```python
from build123d import *

# Parameters (mm, degrees)
ESQUISSE1_W                  = 55
ESQUISSE1_H                  = 45
BOSS_EXTRU_1_DEPTH           = 12
ESQUISSE2_R                  = 4.25
ENL_V_MAT_EXTRU_1_DEPTH      = 55.085580333
ENL_V_MAT_EXTRU_2_DEPTH      = 12.25
ENL_V_MAT_EXTRU_2_DEPTH_BACK = 12.25
ESQUISSE3_R                  = 7.75
ESQUISSE4_R                  = 11
ENL_V_MAT_EXTRU_3_DEPTH      = 3
ESQUISSE5_R                  = 5
ENL_V_MAT_EXTRU_4_DEPTH      = 15
ENL_V_MAT_EXTRU_5_DEPTH      = 38.503333185
ENL_V_MAT_EXTRU_5_DEPTH_BACK = 38.503333185
ESQUISSE6_R                  = 1.5
ESQUISSE7_R                  = 2.5
ENL_V_MAT_EXTRU_6_DEPTH      = 4
CHANFREIN3_SIZE              = 5
ESQUISSE9_W                  = 60
ESQUISSE9_H                  = 18
BOSS_EXTRU_2_DEPTH           = 25
ESQUISSE10_W                 = 40.5
ESQUISSE10_H                 = 20
ENL_V_MAT_EXTRU_7_DEPTH      = 30
ESQUISSE11_R                 = 2.15
ENL_V_MAT_EXTRU_8_DEPTH      = 51.17220346
CONG_2_R                     = 5
CONG_3_R                     = 5
ESQUISSE12_W                 = 5
ESQUISSE12_H                 = 2
ENL_V_MAT_EXTRU_9_DEPTH      = 9
SYM_TRIE4_COPY_1_SKETCH_W    = 5
SYM_TRIE4_COPY_1_SKETCH_H    = 2
SYM_TRIE4_COPY_1_DEPTH       = 9
ESQUISSE13_W                 = 29
ESQUISSE13_H                 = 3
BOSS_EXTRU_3_DEPTH           = 25
BOSS_EXTRU_4_REACH           = 52.172
ESQUISSE14_W                 = 29
ESQUISSE14_H                 = 2.5
ESQUISSE15_R                 = 1.5
ENL_V_MAT_EXTRU_10_DEPTH     = 9
ENL_V_MAT_EXTRU_11_DEPTH     = 2


with BuildPart() as part:
    # Esquisse1 → Boss.-Extru.1 (new body)
    with BuildSketch(Plane.XY):
        Rectangle(ESQUISSE1_W, ESQUISSE1_H)
    extrude(amount=BOSS_EXTRU_1_DEPTH)

    # Esquisse2 → Enlèv. mat.-Extru.1 (cut, through all)
    with BuildSketch(Plane(origin=(0, 22.5, 0), x_dir=(1, 0, 0), z_dir=(0, 1, 0))):
        with Locations((-12.5, -12)):
            Circle(ESQUISSE2_R)
        with Locations((12.5, -12)):
            Circle(ESQUISSE2_R)
    extrude(amount=-ENL_V_MAT_EXTRU_1_DEPTH, mode=Mode.SUBTRACT)

    # Esquisse3 → Enlèv. mat.-Extru.2 (cut, two sides: drawn at the far end of the back side and taken through both)
    with BuildSketch(Plane(origin=(0, 0, 0), x_dir=(1, 0, 0), z_dir=(0, 1, 0)).offset(-ENL_V_MAT_EXTRU_2_DEPTH_BACK)):
        with Locations((-12.5, -12)):
            Circle(ESQUISSE3_R)
    extrude(amount=ENL_V_MAT_EXTRU_2_DEPTH + ENL_V_MAT_EXTRU_2_DEPTH_BACK, mode=Mode.SUBTRACT)

    # Esquisse4 → Enlèv. mat.-Extru.3 (cut)
    with BuildSketch(Plane(origin=(0, 7.5, 0), x_dir=(1, 0, 0), z_dir=(0, 1, 0))):
        with Locations((12.5, -12)):
            Circle(ESQUISSE4_R)
    enl_v_mat_extru_3 = extrude(amount=-ENL_V_MAT_EXTRU_3_DEPTH, mode=Mode.SUBTRACT)

    # Esquisse5 → Enlèv. mat.-Extru.4 (cut)
    with BuildSketch(Plane(origin=(0, 7.5, 0), x_dir=(1, 0, 0), z_dir=(0, 1, 0))):
        with Locations((12.5, -12)):
            Circle(ESQUISSE5_R)
    extrude(amount=-ENL_V_MAT_EXTRU_4_DEPTH, mode=Mode.SUBTRACT)

    # Esquisse6 → Enlèv. mat.-Extru.5 (cut, two sides: drawn at the far end of the back side and taken through both)
    with BuildSketch(Plane(origin=(0, 0, 0), x_dir=(-1, 0, 0), z_dir=(0, 0, -1)).offset(-ENL_V_MAT_EXTRU_5_DEPTH_BACK)):
        with Locations((23.5, -18.5)):
            Circle(ESQUISSE6_R)
        with Locations((-23.5, -18.5)):
            Circle(ESQUISSE6_R)
        with Locations((-23.5, 18.5)):
            Circle(ESQUISSE6_R)
        with Locations((23.5, 18.5)):
            Circle(ESQUISSE6_R)
    extrude(amount=ENL_V_MAT_EXTRU_5_DEPTH + ENL_V_MAT_EXTRU_5_DEPTH_BACK, mode=Mode.SUBTRACT)

    # Esquisse7 → Enlèv. mat.-Extru.6 (cut)
    with BuildSketch(Plane(origin=(0, 0, 0), x_dir=(-1, 0, 0), z_dir=(0, 0, -1))):
        with Locations((23.5, -18.5)):
            Circle(ESQUISSE7_R)
        with Locations(Location((23.5, 18.5, 0), (0, 0, 180))):
            Circle(ESQUISSE7_R)
        with Locations((-23.5, 18.5)):
            Circle(ESQUISSE7_R)
        with Locations(Location((-23.5, -18.5, 0), (0, 0, 180))):
            Circle(ESQUISSE7_R)
    extrude(amount=-ENL_V_MAT_EXTRU_6_DEPTH, mode=Mode.SUBTRACT)

    # Chanfrein3
    # the kernel refuses this chamfer: 5 mm, written as the material it takes off along each edge
    with BuildSketch(Plane(origin=(-27.5, 35.35841494, 0), x_dir=(0.9996219169112968, 0, -0.027495876610586372), z_dir=(0, -1, 0)), Plane(origin=(27.5, -35.35841494, 0), x_dir=(-0.9996219169112968, 0, -0.027495876610586372), z_dir=(0, 1, 0))) as chanfrein3_piece_1:
        Polygon((CHANFREIN3_SIZE * 0.999621916911, CHANFREIN3_SIZE * 0.0274958766106), (-CHANFREIN3_SIZE * 0.0274958766106, CHANFREIN3_SIZE * 0.999621916911), (0, 0), align=None)
    extrude(amount=70.71682988, mode=Mode.SUBTRACT)

    # Symétrie2: Enlèv. mat.-Extru.3 across plane
    add(enl_v_mat_extru_3.mirror(Plane.ZX), mode=Mode.SUBTRACT)

    # Esquisse9 → Boss.-Extru.2 (add)
    with BuildSketch(Plane(origin=(0, 0, 0), x_dir=(-1, 0, 0), z_dir=(0, 0, -1))):
        Rectangle(ESQUISSE9_W, ESQUISSE9_H)
    extrude(amount=BOSS_EXTRU_2_DEPTH)

    # Esquisse10 → Enlèv. mat.-Extru.7 (cut)
    with BuildSketch(Plane(origin=(0, 9, 0), x_dir=(1, 0, 0), z_dir=(0, 1, 0))):
        with Locations((0, 12.5)):
            Rectangle(ESQUISSE10_W, ESQUISSE10_H)
    extrude(amount=-ENL_V_MAT_EXTRU_7_DEPTH, mode=Mode.SUBTRACT)

    # Esquisse11 → Enlèv. mat.-Extru.8 (cut, through all)
    with BuildSketch(Plane(origin=(0, -9, 0), x_dir=(-1, 0, 0), z_dir=(0, -1, 0))):
        with Locations(Location((-23.65, 7.4, 0), (0, 0, 90))):
            Circle(ESQUISSE11_R)
        with Locations(Location((-23.65, 17.6, 0), (0, 0, 90))):
            Circle(ESQUISSE11_R)
        with Locations(Location((24.15, 7.4, 0), (0, 0, 90))):
            Circle(ESQUISSE11_R)
        with Locations(Location((24.15, 17.6, 0), (0, 0, 90))):
            Circle(ESQUISSE11_R)
    extrude(amount=-ENL_V_MAT_EXTRU_8_DEPTH, mode=Mode.SUBTRACT)

    # Congé2
    cong_2_edges = [part.edges().sort_by_distance(p)[0] for p in [
        (-30, 0, 0),
        (30, 0, 0),
    ]]
    fillet(cong_2_edges, radius=CONG_2_R)

    # Congé3
    cong_3_edges = [part.edges().sort_by_distance(p)[0] for p in [
        (-30, 0, -25),
        (30, 0, -25),
    ]]
    fillet(cong_3_edges, radius=CONG_3_R)

    # Esquisse12 → Enlèv. mat.-Extru.9 (cut)
    with BuildSketch(Plane(origin=(30, 0, 0), x_dir=(0, 0, -1), z_dir=(1, 0, 0))):
        with Locations((7.4, 4.5)):
            Rectangle(ESQUISSE12_W, ESQUISSE12_H)
        with Locations((17.6, 4.5)):
            Rectangle(ESQUISSE12_W, ESQUISSE12_H)
    enl_v_mat_extru_9 = extrude(amount=-ENL_V_MAT_EXTRU_9_DEPTH, mode=Mode.SUBTRACT)

    # Symétrie3: Enlèv. mat.-Extru.9 across plane
    add(enl_v_mat_extru_9.mirror(Plane(origin=(0, 0, 0), x_dir=(0, 0, 1), z_dir=(1, 0, 0))), mode=Mode.SUBTRACT)

    # Symétrie4: Enlèv. mat.-Extru.9 across plane
    add(enl_v_mat_extru_9.mirror(Plane.ZX), mode=Mode.SUBTRACT)

    # Symétrie4 copy 1 sketch → Symétrie4 copy 1 (cut)
    with BuildSketch(Plane(origin=(-30, 0, 0), x_dir=(0, 0, -1), z_dir=(-1, 0, 0))):
        with Locations((7.4, 4.5)):
            Rectangle(SYM_TRIE4_COPY_1_SKETCH_W, SYM_TRIE4_COPY_1_SKETCH_H)
        with Locations((17.6, 4.5)):
            Rectangle(SYM_TRIE4_COPY_1_SKETCH_W, SYM_TRIE4_COPY_1_SKETCH_H)
    extrude(amount=-SYM_TRIE4_COPY_1_DEPTH, mode=Mode.SUBTRACT)

    # Esquisse13 → Boss.-Extru.3 (add)
    with BuildSketch(Plane(origin=(0, 0, 0), x_dir=(-1, 0, 0), z_dir=(0, 0, -1))):
        with Locations((0, 21)):
            Rectangle(ESQUISSE13_W, ESQUISSE13_H)
    extrude(amount=BOSS_EXTRU_3_DEPTH)

    # Esquisse14 → Boss.-Extru.4 (add, up to next)
    with BuildSketch(Plane(origin=(0, 9, 0), x_dir=(1, 0, 0), z_dir=(0, 1, 0)), mode=Mode.PRIVATE) as boss_extru_4_sk1:
        with Locations((0, 23.75)):
            Rectangle(ESQUISSE14_W, ESQUISSE14_H)
    boss_extru_4_tool1 = extrude(boss_extru_4_sk1.sketch, amount=BOSS_EXTRU_4_REACH, mode=Mode.PRIVATE) - part.part
    add(boss_extru_4_tool1.solids().sort_by_distance((0, 9, -23.75))[0])

    # Esquisse15 → Enlèv. mat.-Extru.10 (cut)
    with BuildSketch(Plane(origin=(0, 22.5, 0), x_dir=(1, 0, 0), z_dir=(0, 1, 0))):
        with Locations(Location((-10.25, 12.5, 0), (0, 0, 270))):
            Circle(ESQUISSE15_R)
    extrude(amount=-ENL_V_MAT_EXTRU_10_DEPTH, mode=Mode.SUBTRACT)

    # Esquisse16 → Enlèv. mat.-Extru.11 (cut)
    with BuildSketch(Plane(origin=(0, 22.5, 0), x_dir=(1, 0, 0), z_dir=(0, 1, 0))):
        Polygon((-8.806624327, 15), (-11.693375673, 15), (-13.136751346, 12.5), (-11.693375673, 10), (-8.806624327, 10), (-7.363248654, 12.5), align=None)
    extrude(amount=-ENL_V_MAT_EXTRU_11_DEPTH, mode=Mode.SUBTRACT)


solid = part.part
```
Part model, mm, in its own coordinate system. A direction names the side the tool comes from. Round coordinates to 2 decimals unless told otherwise and drop trailing zeros. Write each loop counter-clockwise with the first axis right and the second up, starting at its lowest first coordinate (ties: lowest second). Pieces come first, ordered by that corner, then holes. Notation, with made-up numbers: M -19.75,73.25 L -6.75,73.25 A23 cw -6.75,90.25 Z; hole C -13,83.25 d5. An arc over 180 degrees is marked long. Answer as CSV lines item,"result". Start each with the question number.
1) Band-saw the part on C-C (x = -4). List the corners of the cut face in (y, z), then the cut area to 3 significant figures.
2) Drill centre lines: L1, parallel to Y at x = 23.5, z = 10.5; L2, parallel to X at y = 0.5, z = -7.4; L3, parallel to Y at x = -27, z = -19.5. Where is each one in solid material? Low to high.
3) Drop flat-ended pins along their axis: pin 1 (5.5 mm diameter, centred on x = 24, y = -17.5, fed in from -Z); pin 2 (5 mm diameter, centred on x = 12.5, y = -6, fed in from +Z); pin 3 (5.5 mm diameter, centred on x = 23.65, z = -7.4, fed in from +Y); pin 4 (2.5 mm diameter, centred on x = 24.5, z = -7.5, fed in from +Y). Give the stop position or say it passes through.
4) Band-saw the part on A-A (y = 14). List the corners of the cut face in (x, z), then the cut area to 3 significant figures.
5) Band-saw the part on B-B (y = 6.5). List the corners of the cut face in (x, z).
6) Which spindle directions (+Z, -Z, +X, -X, +Y, -Y) get a long thin tool onto all of the face, cutting with end or side? Do faces 1 (the face through (-22, 20, 4)), 2 (the face through (-27, 5.5, -18)), 3 (the face through (14.5, 20, -15)). Say none if no direction does.
7) Band-saw the part on D-D (y = 18.5). List the corners of the cut face in (x, z), then the cut area to 3 significant figures.
8) Mould opens along X. For faces 4 (the face through (-22.39, -17.49, 8.06)), 5 (the face through (-26, -4, -15.1)), 6 (the face through (-22.34, -0.05, -18.76)), 7 (the face through (27.5, 0, 8)) say: +X half, -X half, draft (parallel to the pull), parting line (faces both ways), or undercut.
Worked out:
1,outline,"M -22.5,0 L -9,0 L -9,-2.5 L 9,-2.5 L 9,0 L 19.5,0 L 19.5,-22.5 L -9,-22.5 L -9,-25 L 22.5,-25 L 22.5,12 L -22.5,12 Z"
1,area,"731 mm²"
2,L1,"-22.5 to -20, -17 to 17, 20 to 22.5"
2,L2,"-30 to -26.3, -22 to -20.25, 20.25 to 21.5, 25.8 to 30"
2,L3,"-9 to -5.5, -3.5 to 3.5, 5.5 to 9"
3,pin 1,"z = 0"
3,pin 2,"z = 8.25"
3,pin 3,"y = 9"
3,pin 4,"through"
4,outline,"M -27.5,5 L -22.5,0 L 22.5,0 L 27.5,5 L 27.5,12 L 16.75,12 A4.25 cw 8.25,12 L -8.25,12 A4.25 cw -16.75,12 L -27.5,12 Z; M -14.5,-25 L 14.5,-25 L 14.5,-22.5 L -14.5,-22.5 Z"
4,area,"651 mm²"
5,outline,"M -30,-20 A5 ccw -25,-25 L 25,-25 A5 ccw 30,-20 L 30,-5 A5 ccw 25,0 L 22.5,0 L 27.5,5 L 27.5,12 L 23.5,12 A11 cw 1.5,12 L -4.75,12 A7.75 cw -20.25,12 L -27.5,12 L -27.5,5 L -22.5,0 L -25,0 A5 ccw -30,-5 Z; hole C -24.15,-17.6 d4.3; hole C -24.15,-7.4 d4.3; hole M -20.25,-22.5 L 20.25,-22.5 L 20.25,-2.5 L -20.25,-2.5 Z; hole C 23.65,-17.6 d4.3; hole C 23.65,-7.4 d4.3"
6,face 1,"-Z"
6,face 2,"-X"
6,face 3,"-Z, +X, +Y"
7,outline,"M -27.5,5 L -26,3.5 L -26,4 L -25,4 L -25,12 L -27.5,12 Z; M -22,4 L -21,4 L -21,0 L 21,0 L 21,4 L 22,4 L 22,12 L 16.75,12 A4.25 cw 8.25,12 L -8.25,12 A4.25 cw -16.75,12 L -22,12 Z; M -14.5,-25 L 14.5,-25 L 14.5,-22.5 L -14.5,-22.5 Z; M 25,4 L 26,4 L 26,3.5 L 27.5,5 L 27.5,12 L 25,12 Z"
7,area,"575 mm²"
8,face 4,"undercut"
8,face 5,"draft"
8,face 6,"undercut"
8,face 7,"+X half"
